For this review, take the finished solid that the model builds, in its own axes (mm). A direction names the side the tool comes from. Coordinates: 2 decimals unless noted, no trailing zeros. Loops run counter-clockwise (first coordinate to the right, second up) from the corner with the lowest first, then second, coordinate; pieces in that order, holes last. Notation, with made-up numbers: (58.5, 78.5) -> (96.5, 78.5) arc R20 ccw to (96.5, 94.5) -> close; hole circle Ø6 at (62, -38.75). An arc over 180 degrees is marked (long way). Answer in a Markdown table with one row per item.
from build123d import *

# Parameters (mm, degrees)
SKETCH1_R                                       = 43
BASE_DEPTH                                      = 3
M4_CLEARANCE_HOLE1_D                            = 4.5
M4_CLEARANCE_HOLE2_D                            = 6.35
F_1_4_CLEARANCE_HOLE1_D                         = 6.7564
FILLET1_R                                       = 10
CSK_FOR_M4_FLAT_HEAD_MACHINE_SCREW1_D           = 4.5
CSK_FOR_M4_FLAT_HEAD_MACHINE_SCREW1_CSINK_D     = 9.4
CSK_FOR_M4_FLAT_HEAD_MACHINE_SCREW1_CSINK_ANGLE = 90
SKETCH15_R                                      = 4.165
CUT_EXTRUDE1_DEPTH                              = 134.200037538


with BuildPart() as part:
    # Sketch1 → base (new, symmetric)
    with BuildSketch(Plane.XY):
        with BuildLine():
            Line((-36, 44.83581158), (-36, 120))
            Line((-36, 120), (36, 120))
            Line((36, 120), (36, 44.83581158))
            ThreePointArc((36, 44.83581158), (0, -57.5), (-36, 44.83581158))
        make_face()
        Circle(SKETCH1_R, mode=Mode.SUBTRACT)
    extrude(amount=BASE_DEPTH, both=True)

    # M4 Clearance Hole1 (through all)
    with Locations(Plane.XY.offset(3)):
        with Locations((0, 50), (25, 43.301270189), (43.301270189, 25), (50, 0), (43.301270189, -25), (25, -43.301270189), (0, -50), (-25, -43.301270189), (-43.301270189, -25), (-50, 0), (-43.301270189, 25), (-25, 43.301270189)):
            Hole(M4_CLEARANCE_HOLE1_D / 2)

    # M4 Clearance Hole2 (through all)
    with Locations(Plane.XY.offset(3)):
        with Locations((0, 60), (0, 110.8)):
            Hole(M4_CLEARANCE_HOLE2_D / 2)

    # 1/4 Clearance Hole1 (through all)
    with Locations(Plane.XY.offset(3)):
        with Locations((-12.7, 85.4), (12.7, 85.4)):
            Hole(F_1_4_CLEARANCE_HOLE1_D / 2)

    # Fillet1
    fillet1_edges = [part.edges().sort_by_distance(p)[0] for p in [
        (-36, 44.83581158, 0),
        (-36, 120, 0),
        (36, 120, 0),
        (36, 44.83581158, 0),
    ]]
    fillet(fillet1_edges, radius=FILLET1_R)

    # CSK for M4 Flat Head Machine Screw1 (through all)
    with Locations(Plane.XY.offset(3)):
        with Locations((0, 50), (25, 43.301270189), (43.301270189, 25), (50, 0), (43.301270189, -25), (25, -43.301270189), (0, -50), (-25, -43.301270189), (-43.301270189, -25), (-50, 0), (-43.301270189, 25), (-25, 43.301270189)):
            CounterSinkHole(CSK_FOR_M4_FLAT_HEAD_MACHINE_SCREW1_D / 2, CSK_FOR_M4_FLAT_HEAD_MACHINE_SCREW1_CSINK_D / 2, counter_sink_angle=CSK_FOR_M4_FLAT_HEAD_MACHINE_SCREW1_CSINK_ANGLE)

    # Sketch15 → Cut-Extrude1 (cut, through all)
    with BuildSketch(Plane(origin=(0, 0, -3), x_dir=(-1, 0, 0), z_dir=(0, 0, -1))):
        with Locations((22.335, 108.435)):
            Circle(SKETCH15_R)
    extrude(amount=-CUT_EXTRUDE1_DEPTH, mode=Mode.SUBTRACT)


solid = part.part
Item 1: Take a section at A-A, the plane x = 0. State the section outline as (y, z) points (3 decimals), and give its area (3 significant figures).
Worked answers:
| item | result |
|---|---|
| outline | (-57.5, -3) -> (-52.25, -3) -> (-52.25, 0.55) -> (-54.7, 3) -> (-57.5, 3) -> close; (-47.75, -3) -> (-43, -3) -> (-43, 3) -> (-45.3, 3) -> (-47.75, 0.55) -> close; (43, -3) -> (47.75, -3) -> (47.75, 0.55) -> (45.3, 3) -> (43, 3) -> close; (52.25, -3) -> (56.825, -3) -> (56.825, 3) -> (54.7, 3) -> (52.25, 0.55) -> close; (63.175, -3) -> (107.625, -3) -> (107.625, 3) -> (63.175, 3) -> close; (113.975, -3) -> (120, -3) -> (120, 3) -> (113.975, 3) -> close |
| area | 407 mm² |
Item 2: The part is to be moulded in two halves that separate along X. For faces 3 (the cylindrical face through (-5.598, 42.634, -0.042)), 4 (the cylindrical face through (-36.81, 45.46, 0.04)), 5 (the flat face through (36, 80, 0)), say which applies: +X half, -X half, draft (parallel to the pull), parting line (faces both ways), or undercut.
Worked answers:
| item | result |
|---|---|
| face 3 | undercut |
| face 4 | -X half |
| face 5 | +X half |
Item 3: Take a section at C-C, the plane x = -12.7. State the section outline as (y, z) points.
Worked answers:
| item | result |
|---|---|
| outline | (-56.08, -3) -> (-41.08, -3) -> (-41.08, 3) -> (-56.08, 3) -> close; (41.08, -3) -> (82.02, -3) -> (82.02, 3) -> (41.08, 3) -> close; (88.78, -3) -> (120, -3) -> (120, 3) -> (88.78, 3) -> close |
Item 4: For L1, parallel to X at y = 27, z = 1.7; L2, parallel to X at y = -25, z = -0.35; L3, parallel to Y at x = -11, z = -1.75, list the stretches that pass through material, from the lowest coordinate up.
Worked answers:
| item | result |
|---|---|
| L1 | -50.77 to -46.05, -40.55 to -33.47, 33.47 to 40.55, 46.05 to 50.77 |
| L2 | -51.78 to -45.55, -41.05 to -34.99, 34.99 to 41.05, 45.55 to 51.78 |
| L3 | -56.44 to -41.57, 41.57 to 82.48, 88.32 to 120 |
Item 5: Insertion check: pin 1 (2.5 mm diameter, centred on x = 43.3, y = 25, fed in from -Z); pin 2 (3 mm diameter, centred on y = 89, z = -0.5, fed in from -X); pin 3 (3 mm diameter, centred on y = 47.5, z = -1.5, fed in from +X); pin 4 (5 mm diameter, centred on x = 50, y = 0, fed in from +Z). Each pin has a flat end and moves straight along its axis. Give the tip position at first contact, or say it passes through.
Worked answers:
| item | result |
|---|---|
| pin 1 | through |
| pin 2 | x = -36 |
| pin 3 | x = 36.6 |
| pin 4 | z = 0.8 |
Item 6: For faces 1 (the cylindrical face through (-24.26, 104.74, -0.04)), 2 (the flat face through (-36, 79, 0)), list the 3-axis set-ups (+Z, -Z, +X, -X, +Y, -Y) from which the entire face can be reached by the end or side of a thin tool; tool diameter is ignored.
Worked answers:
| item | result |
|---|---|
| face 1 | +Z, -Z |
| face 2 | +Z, -Z, -X, +Y |
Item 7: Take a section at D-D, the plane z = 1.9. Count the separate pieces of the cut face and the enclosed holes in it, and give its area (3 significant figures).
Worked answers:
| item | result |
|---|---|
| separate pieces | 1 |
| enclosed holes | 18 |
| area | 8,650 mm² |
Item 8: Take a section at B-B, the plane y = -15. State the section outline as (x, z) points.
Worked answers:
| item | result |
|---|---|
| outline | (-55.51, -3) -> (-40.3, -3) -> (-40.3, 3) -> (-55.51, 3) -> close; (40.3, -3) -> (55.51, -3) -> (55.51, 3) -> (40.3, 3) -> close |
